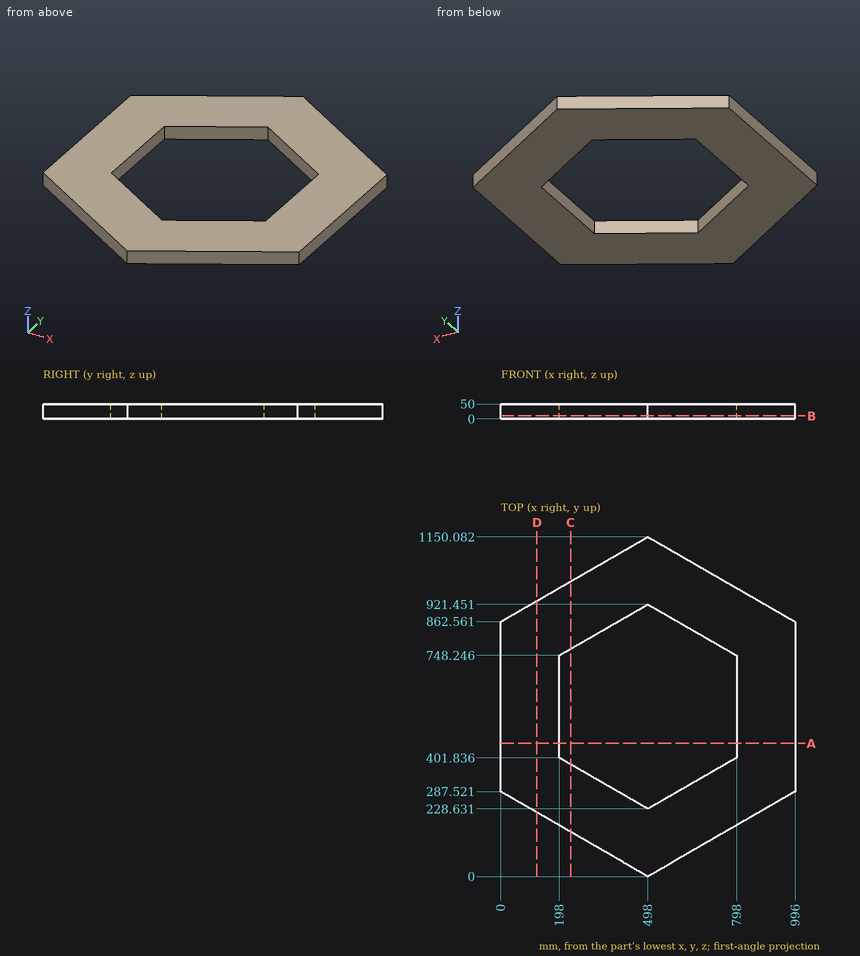
Geometry: see drawing. Coordinates: mm, zero at the bounding-box minimum. Coordinates: 2 decimals unless noted, no trailing zeros. Loops run counter-clockwise (first coordinate to the right, second up) from the corner with the lowest first, then second, coordinate; pieces in that order, holes last.
Q1. Cut plane C-C (x = 236.5). Output: boundary loops of the cut face in (y, z) (1 decimal), then the cut area to 3 significant figures.
Q2. Cut plane A-A (y = 451). Output: boundary loops of the cut face in (x, z).
Q3. Cut plane D-D (x = 122). Output: boundary loops of the cut face in (y, z), then the cut area to 3 significant figures.
Q4. Contact query for flat-ended pins moving along their axis: pin 1 (1 mm diameter, centred on y = 256.5, z = 22.5, fed in from +X) (1 decimal); pin 2 (2 mm diameter, centred on x = 139.5, z = 28.5, fed in from +Y); pin 3 (2 mm diameter, centred on y = 846, z = 7.5, fed in from -X); pin 4 (10 mm diameter, centred on x = 759.5, z = 44, fed in from -Y). Output: stop coordinate, or through.
Q5. Material intervals for line 1 (X direction, y = 607, z = 29); line 2 (X direction, y = 772, z = 30) (1 decimal); line 3 (Y direction, x = 240.5, z = 22.5) (1 decimal), sorted ascending.
Q6. Cut plane B-B (z = 10). Output: boundary loops of the cut face in (x, y) (1 decimal).
Working result:
1. outline: (151, 0) - (379.6, 0) - (379.6, 50) - (151, 50) - close; (770.5, 0) - (999.1, 0) - (999.1, 50) - (770.5, 50) - close
1. area: 22,900 mm2
2. outline: (0, 0) - (198, 0) - (198, 50) - (0, 50) - close; (798, 0) - (996, 0) - (996, 50) - (798, 50) - close
3. outline: (217.08, 0) - (933, 0) - (933, 50) - (217.08, 50) - close
3. area: 35,800 mm2
4. pin 1: stops at x = 943.1
4. pin 2: stops at y = 943.68
4. pin 3: stops at x = 0
4. pin 4: stops at y = 148.09
5. line 1: x = 0 to 198, 798 to 996
5. line 2: x = 0 to 239.1, 756.9 to 996
5. line 3: y = 148.7 to 377.3, 772.8 to 1001.4
6. outline: (0, 287.5) - (498, 0) - (996, 287.5) - (996, 862.6) - (498, 1150.1) - (0, 862.6) - close; hole (198, 401.8) - (498, 228.6) - (798, 401.8) - (798, 748.2) - (498, 921.5) - (198, 748.2) - close
